from build123d import *

# Parameters (mm, degrees)
SKETCH1_W                = 76.2
SKETCH1_H                = 51
BOSS_EXTRUDE1_DEPTH      = 10
CHAMFER1_SIZE            = 2
BOSS_EXTRUDE2_DEPTH      = 38.1
BOSS_EXTRUDE2_DEPTH_BACK = 38.1
SKETCH2_W                = 32
SKETCH2_H                = 4.75
CUT_EXTRUDE1_DEPTH       = 32
FILLET1_R                = 13.5
SKETCH4_R                = 4
CUT_EXTRUDE2_DEPTH       = 10
BOSS_EXTRUDE4_START      = -9.1
SKETCH5_W                = 13.5
SKETCH5_H                = 18.25
BOSS_EXTRUDE4_DEPTH      = 8
BOSS_EXTRUDE5_START      = -67.1
SKETCH5_4_W              = 13.5
SKETCH5_4_H              = 18.25
BOSS_EXTRUDE5_DEPTH      = 8
FILLET2_R                = 11.5
BOSS_EXTRUDE6_START      = -9.64
SKETCH7_W                = 13.5
SKETCH7_H                = 10
BOSS_EXTRUDE6_DEPTH      = 6.5
BOSS_EXTRUDE7_START      = -32.36
SKETCH7_2_W              = 13.5
SKETCH7_2_H              = 10
BOSS_EXTRUDE7_DEPTH      = 6.65
FILLET3_R                = 11.5
CHAMFER3_SIZE            = 2
CHAMFER4_SIZE            = 1
SKETCH8_R                = 3.5
SKETCH8_R_2              = 1.8
CUT_EXTRUDE3_DEPTH       = 4.5
SKETCH8_4_R              = 1.8
CUT_EXTRUDE6_DEPTH       = 56.909391028
LPATTERN1_COUNT          = 2
LPATTERN1_PITCH          = 45
SKETCH10_6_R             = 1.8
CUT_EXTRUDE17_DEPTH      = 51.851352048
SKETCH10_R               = 3.5
SKETCH10_R_2             = 1.8
CUT_EXTRUDE11_DEPTH      = 3
SKETCH12_R               = 1.8
CUT_EXTRUDE13_DEPTH      = 56.909391028
SKETCH12_4_R             = 3.5
SKETCH12_4_R_2           = 1.8
CUT_EXTRUDE14_DEPTH      = 4.5
LPATTERN3_COUNT          = 2
LPATTERN3_PITCH          = 50
CUT_EXTRUDE18_DEPTH      = 71.73817429
CUT_EXTRUDE18_DEPTH_BACK = 2.5
SKETCH13_W               = 35
SKETCH13_H               = 12
FILLET4_R                = 8.5
CUT_EXTRUDE19_DEPTH      = 68.931380819
CUT_EXTRUDE19_DEPTH_BACK = 1.5
SKETCH14_R               = 3.5
SKETCH14_R_2             = 1.8
CUT_EXTRUDE20_DEPTH      = 68.931380875
CUT_EXTRUDE20_DEPTH_BACK = 68.931380875
SKETCH14_4_R             = 1.8


with BuildPart() as part:
    # Sketch1 → Boss-Extrude1 (new body)
    with BuildSketch(Plane.XY):
        Rectangle(SKETCH1_W, SKETCH1_H)
    extrude(amount=-BOSS_EXTRUDE1_DEPTH)

    # Chamfer1
    chamfer1_edges = [part.edges().sort_by_distance(p)[0] for p in [
        (-38.1, 25.5, -5),
        (38.1, 25.5, -5),
    ]]
    chamfer(chamfer1_edges, length=CHAMFER1_SIZE)

    # Sketch2 → Boss-Extrude2 (add, two sides: drawn at the far end of the back side and taken through both)
    with BuildSketch(Plane(origin=(0, 0, 0), x_dir=(0, 0, -1), z_dir=(1, 0, 0)).offset(-BOSS_EXTRUDE2_DEPTH_BACK)):
        with Locations((16, -23.125)):
            Rectangle(SKETCH2_W, SKETCH2_H)
    extrude(amount=BOSS_EXTRUDE2_DEPTH + BOSS_EXTRUDE2_DEPTH_BACK)

    # Sketch3 → Cut-Extrude1 (cut)
    with BuildSketch(Plane(origin=(0, -25.5, 0), x_dir=(-1, 0, 0), z_dir=(0, -1, 0))):
        Polygon((-7.67217, 0), (7.67217, 0), (9.268805, 5.32212), (-9.268805, 5.32212), align=None)
    extrude(amount=-CUT_EXTRUDE1_DEPTH, mode=Mode.SUBTRACT)

    # Fillet1
    fillet1_edges = [part.edges().sort_by_distance(p)[0] for p in [
        (0, -20.75, -10),
    ]]
    fillet(fillet1_edges, radius=FILLET1_R)

    # Sketch4 → Cut-Extrude2 (cut)
    with BuildSketch(Plane.XZ.offset(25.5)):
        with Locations((0, -11.5)):
            Circle(SKETCH4_R)
    extrude(amount=-CUT_EXTRUDE2_DEPTH, mode=Mode.SUBTRACT)

    # Sketch5 → Boss-Extrude4 (add)
    with BuildSketch(Plane(origin=(38.1, 0, 0), x_dir=(0, 0, -1), z_dir=(1, 0, 0)).offset(BOSS_EXTRUDE4_START)):
        with Locations((16.75, -11.625)):
            Rectangle(SKETCH5_W, SKETCH5_H)
    extrude(amount=-BOSS_EXTRUDE4_DEPTH)

    # Sketch5<4> → Boss-Extrude5 (add)
    with BuildSketch(Plane(origin=(38.1, 0, 0), x_dir=(0, 0, -1), z_dir=(1, 0, 0)).offset(BOSS_EXTRUDE5_START)):
        with Locations((16.75, -11.625)):
            Rectangle(SKETCH5_4_W, SKETCH5_4_H)
    extrude(amount=BOSS_EXTRUDE5_DEPTH)

    # Fillet2
    fillet2_edges = [part.edges().sort_by_distance(p)[0] for p in [
        (25, -2.5, -10),
        (-25, -2.5, -10),
    ]]
    fillet(fillet2_edges, radius=FILLET2_R)

    # Sketch7 → Boss-Extrude6 (add)
    with BuildSketch(Plane(origin=(21, 0, 0), x_dir=(0, 0, -1), z_dir=(1, 0, 0)).offset(BOSS_EXTRUDE6_START)):
        with Locations((16.75, 4)):
            Rectangle(SKETCH7_W, SKETCH7_H)
    extrude(amount=-BOSS_EXTRUDE6_DEPTH)

    # Sketch7<2> → Boss-Extrude7 (add)
    with BuildSketch(Plane(origin=(21, 0, 0), x_dir=(0, 0, -1), z_dir=(1, 0, 0)).offset(BOSS_EXTRUDE7_START)):
        with Locations((16.75, 4)):
            Rectangle(SKETCH7_2_W, SKETCH7_2_H)
    extrude(amount=BOSS_EXTRUDE7_DEPTH)

    # Fillet3
    # the kernel refuses this fillet: 11.5 mm, written as the material it adds along each edge
    with BuildSketch(Plane(origin=(11.36, -1, -10), x_dir=(0, -1, 0), z_dir=(-1, 0, 0))) as fillet3_piece_1:
        with BuildLine():
            CenterArc((FILLET3_R, -FILLET3_R), FILLET3_R, 90, 90)
            Line((0, -FILLET3_R), (0, 0))
            Line((0, 0), (FILLET3_R, 0))
        make_face()
    extrude(amount=6.5)
    with BuildSketch(Plane(origin=(11.36, -1, -10), x_dir=(0, -1, 0), z_dir=(-1, 0, 0))) as fillet3_piece_2_section:
        with BuildLine():
            CenterArc((FILLET3_R, -FILLET3_R), FILLET3_R, 90, 90)
            Line((0, -FILLET3_R), (0, 0))
            Line((0, 0), (FILLET3_R, 0))
        make_face()
    fillet3_piece_2 = extrude(amount=35.25, mode=Mode.PRIVATE)
    fillet3_piece_2 = split(fillet3_piece_2, bisect_by=Plane(origin=(-4.71, -3.603543814, -12.603543814), z_dir=(-1, 0, 0)), keep=Keep.TOP, mode=Mode.PRIVATE)
    fillet3_piece_2 = split(fillet3_piece_2, bisect_by=Plane(origin=(-11.36, -3.603543814, -12.603543814), z_dir=(1, 0, 0)), keep=Keep.TOP, mode=Mode.PRIVATE)
    add(fillet3_piece_2)
    with BuildSketch(Plane(origin=(-11.36, -1, -10), x_dir=(0, -1, 0), z_dir=(1, 0, 0))) as fillet3_piece_3:
        with BuildLine():
            CenterArc((FILLET3_R, FILLET3_R), FILLET3_R, 180, 90)
            Line((0, FILLET3_R), (0, 0))
            Line((0, 0), (FILLET3_R, 0))
        make_face()
    extrude(amount=6.65)
    with BuildSketch(Plane(origin=(-11.36, -1, -10), x_dir=(0, -1, 0), z_dir=(1, 0, 0))) as fillet3_piece_4_section:
        with BuildLine():
            CenterArc((FILLET3_R, FILLET3_R), FILLET3_R, 180, 90)
            Line((0, FILLET3_R), (0, 0))
            Line((0, 0), (FILLET3_R, 0))
        make_face()
    fillet3_piece_4 = extrude(amount=35.4, mode=Mode.PRIVATE)
    fillet3_piece_4 = split(fillet3_piece_4, bisect_by=Plane(origin=(11.36, -3.603543814, -12.603543814), z_dir=(-1, 0, 0)), keep=Keep.TOP, mode=Mode.PRIVATE)
    fillet3_piece_4 = split(fillet3_piece_4, bisect_by=Plane(origin=(4.86, -3.603543814, -12.603543814), z_dir=(1, 0, 0)), keep=Keep.TOP, mode=Mode.PRIVATE)
    add(fillet3_piece_4)

    # Chamfer3
    chamfer3_edges = [part.edges().sort_by_distance(p)[0] for p in [
        (38.1, -23.125, -32),
        (-38.1, -23.125, -32),
    ]]
    chamfer(chamfer3_edges, length=CHAMFER3_SIZE)

    # Chamfer4
    chamfer4_edges = [part.edges().sort_by_distance(p)[0] for p in [
        (-25, -2.5, -23.5),
        (8.11, 9, -23.5),
        (8.11, -1, -23.5),
        (0, 25.5, 0),
        (-8.035, -1, -23.5),
        (-8.035, 9, -23.5),
        (0, 25.5, -10),
        (0, -20.75, -32),
        (25, -2.5, -23.5),
    ]]
    chamfer(chamfer4_edges, length=CHAMFER4_SIZE)

    # Sketch8 → Cut-Extrude3 (cut)
    with BuildSketch(Plane.XY):
        with Locations((-30.63, 21.5)):
            Circle(SKETCH8_R)
        with Locations((-30.63, 21.5)):
            Circle(SKETCH8_R_2, mode=Mode.SUBTRACT)
    cut_extrude3 = extrude(amount=-CUT_EXTRUDE3_DEPTH, mode=Mode.SUBTRACT)

    # Sketch8<4> → Cut-Extrude6 (cut, through all)
    with BuildSketch(Plane.XY):
        with Locations((-30.63, 21.5)):
            Circle(SKETCH8_4_R)
    cut_extrude6 = extrude(amount=-CUT_EXTRUDE6_DEPTH, mode=Mode.SUBTRACT)

    # LPattern1: Cut-Extrude3, Cut-Extrude6 ×2
    with Locations(*[(i * LPATTERN1_PITCH, 0, 0) for i in range(1, LPATTERN1_COUNT)]):
        add(cut_extrude3, mode=Mode.SUBTRACT)
        add(cut_extrude6, mode=Mode.SUBTRACT)

    # Sketch10<6> → Cut-Extrude17 (cut, through all)
    with BuildSketch(Plane.XY.offset(-10)):
        with Locations(Location((-16.6, 6.5, 0), (0, 0, 180))):
            Circle(SKETCH10_6_R)
        with Locations(Location((15.4, 6.5, 0), (0, 0, 180))):
            Circle(SKETCH10_6_R)
    extrude(amount=CUT_EXTRUDE17_DEPTH, mode=Mode.SUBTRACT)

    # Sketch10 → Cut-Extrude11 (cut)
    # profile 1 of 2: a face of its own
    with BuildSketch(Plane.XY.offset(-10)):
        with Locations(Location((-16.6, 6.5, 0), (0, 0, 180))):
            Circle(SKETCH10_R)
        with Locations(Location((-16.6, 6.5, 0), (0, 0, 180))):
            Circle(SKETCH10_R_2, mode=Mode.SUBTRACT)
    # profile 2 of 2: a face of its own
    with BuildSketch(Plane.XY.offset(-10)):
        with Locations(Location((15.4, 6.5, 0), (0, 0, 180))):
            Circle(SKETCH10_R)
        with Locations(Location((15.4, 6.5, 0), (0, 0, 180))):
            Circle(SKETCH10_R_2, mode=Mode.SUBTRACT)
    extrude(amount=CUT_EXTRUDE11_DEPTH, mode=Mode.SUBTRACT)

    # Sketch12 → Cut-Extrude13 (cut, through all)
    with BuildSketch(Plane.XY):
        with Locations((-25, -8.5)):
            Circle(SKETCH12_R)
    cut_extrude13 = extrude(amount=-CUT_EXTRUDE13_DEPTH, mode=Mode.SUBTRACT)

    # Sketch12<4> → Cut-Extrude14 (cut)
    with BuildSketch(Plane.XY):
        with Locations((-25, -8.5)):
            Circle(SKETCH12_4_R)
        with Locations((-25, -8.5)):
            Circle(SKETCH12_4_R_2, mode=Mode.SUBTRACT)
    cut_extrude14 = extrude(amount=-CUT_EXTRUDE14_DEPTH, mode=Mode.SUBTRACT)

    # LPattern3: Cut-Extrude13, Cut-Extrude14 ×2
    with Locations(*[(i * LPATTERN3_PITCH, 0, 0) for i in range(1, LPATTERN3_COUNT)]):
        add(cut_extrude13, mode=Mode.SUBTRACT)
        add(cut_extrude14, mode=Mode.SUBTRACT)

    # Sketch13 → Cut-Extrude18 (cut, two sides: drawn at the far end of the back side and taken through both)
    with BuildSketch(Plane(origin=(0, -20.75, 5.592775926), x_dir=(1, 0, 0), z_dir=(0, 1, 0)).offset(-CUT_EXTRUDE18_DEPTH_BACK)):
        with Locations((0, 31.592775926)):
            Rectangle(SKETCH13_W, SKETCH13_H)
    extrude(amount=CUT_EXTRUDE18_DEPTH + CUT_EXTRUDE18_DEPTH_BACK, mode=Mode.SUBTRACT)

    # Fillet4
    # the kernel refuses this fillet: 8.5 mm, written as the material it adds along each edge
    with BuildSketch(Plane(origin=(33.619877511, -23.25, -20), x_dir=(0, 0, -1), z_dir=(-1, 0, 0))) as fillet4_piece_1:
        with BuildLine():
            CenterArc((6.447951004, -8.5), FILLET4_R, 90, 49.339390538)
            Line((0, -2.96159519), (-0.12895902, -2.850827093))
            ThreePointArc((-0.12895902, -2.850827093), (-0.17, -1.480797595), (-0.17, 0))
            Line((-0.17, 0), (0, 0.17))
            Line((0, 0.17), (6.447951004, 0.17))
            Line((6.447951004, 0.17), (6.447951004, 0))
        make_face()
    extrude(amount=67.239755022)

    # Sketch14 → Cut-Extrude19 (cut, two sides: drawn at the far end of the back side and taken through both)
    # profile 1 of 2: a face of its own
    with BuildSketch(Plane(origin=(0, -20.75, 0), x_dir=(1, 0, 0), z_dir=(0, 1, 0)).offset(-CUT_EXTRUDE19_DEPTH_BACK)):
        with Locations(Location((-33.55, 17, 0), (0, 0, 90))):
            Circle(SKETCH14_R)
        with Locations(Location((-33.55, 17, 0), (0, 0, 90))):
            Circle(SKETCH14_R_2, mode=Mode.SUBTRACT)
    # profile 2 of 2: a face of its own
    with BuildSketch(Plane(origin=(0, -20.75, 0), x_dir=(1, 0, 0), z_dir=(0, 1, 0)).offset(-CUT_EXTRUDE19_DEPTH_BACK)):
        with Locations(Location((33.55, 17, 0), (0, 0, 90))):
            Circle(SKETCH14_R)
        with Locations(Location((33.55, 17, 0), (0, 0, 90))):
            Circle(SKETCH14_R_2, mode=Mode.SUBTRACT)
    extrude(amount=CUT_EXTRUDE19_DEPTH + CUT_EXTRUDE19_DEPTH_BACK, mode=Mode.SUBTRACT)

    # Sketch14<4> → Cut-Extrude20 (cut, two sides: drawn at the far end of the back side and taken through both)
    with BuildSketch(Plane(origin=(0, -20.75, 0), x_dir=(1, 0, 0), z_dir=(0, 1, 0)).offset(-CUT_EXTRUDE20_DEPTH_BACK)):
        with Locations(Location((33.55, 17, 0), (0, 0, 270))):
            Circle(SKETCH14_4_R)
        with Locations(Location((-33.55, 17, 0), (0, 0, 270))):
            Circle(SKETCH14_4_R)
    extrude(amount=CUT_EXTRUDE20_DEPTH + CUT_EXTRUDE20_DEPTH_BACK, mode=Mode.SUBTRACT)


solid = part.part
Could you check a few things on this model? Use its own coordinates, in mm. A direction names the side the tool comes from. Give positions to 0.01 mm unless a question says otherwise; leave off trailing zeros. Write each loop counter-clockwise with the first axis right and the second up, starting at its lowest first coordinate (ties: lowest second). Pieces come first, ordered by that corner, then holes. Notation, with made-up numbers: (56, -3.5) - (110, -3.5) arc R22 ccw to (110, 33.5) - close; hole circle Ø9 at (-22.75, 80). An arc over 180 degrees is marked (long way). Use CSV: the item, a comma, the result in double quotes. Start each with the question number.
Item 1: For faces 1 (the face through (-34, -22.25, -15)), 2 (the face through (16.159, 9.917, -8.521)), 3 (the face through (8.482, -9.724, -2.698)), 4 (the face through (8, 4, -20)), which set-ups out of +Z, -Z, +X, -X, +Y, -Y let a thin tool reach every point of the face, with its end or its side?
Item 2: I want a section at D-D, the plane y = 15. Please give me the cut outline in (x, z), then the cut area to 3 significant figures.
Item 3: I want a section at B-B, the plane z = -25. Please give me the cut outline in (x, y), then the cut area to 3 significant figures.
Item 4: I want a section at C-C, the plane x = 25. Please give me the cut outline in (y, z).
Item 5: If I drill on line 1 along Z through (x, y) = (-33.55, -23.15); line 2 along Y through (x, z) = (-30.63, -7.9); line 3 along X through (y, z) = (-13, -17), over which ranges is the centre line in solid material (lowest first)?
Item 6: If we mould it in two halves opening along Y, with no side actions, what happens to faces 5 (the face through (-29, 20, -4.5)), 6 (the face through (37.1, 24.5, -4.9)), 7 (the face through (-1, 12, -10))? For each: pulls with the +Y half, pulls with the -Y half, needs draft (parallel to the pull), parting line crosses it, or undercut.
Item 7: I'm going to push flat-ended pins straight in: pin 1 (12 mm diameter, centred on y = 4.5, z = -18.5, fed in from +X); pin 2 (4 mm diameter, centred on y = -10, z = -20, fed in from +X); pin 3 (7.5 mm diameter, centred on x = 34.5, z = -17.5, fed in from +Y). Where does each tip first touch, or does it pass through?
Item 8: I want a section at A-A, the plane x = -16.6. Please give me the cut outline in (y, z).
Findings:
1,face 1,"+Y"
1,face 2,"-Z"
1,face 3,"-Y"
1,face 4,"-Z, +X, -X, +Y"
2,outline,"(-38.1, -10) - (38.1, -10) - (38.1, 0) - (-38.1, 0) - close"
2,area,"762 mm2"
3,outline,"(-38.1, -25.5) - (38.1, -25.5) - (38.1, -20.75) - (17.5, -20.75) - (17.5, -23.13) - (-17.5, -23.13) - (-17.5, -20.75) - (-38.1, -20.75) - close"
3,area,"279 mm2"
4,outline,"(-25.5, -32) - (-21.75, -32) - (-20.75, -31) - (-20.75, -23.5) - (-10.3, -23.5) - (-10.3, -4.5) - (-12, -4.5) - (-12, 0) - (-25.5, 0) - close; (-6.7, -23.5) - (-3.5, -23.5) - (-2.5, -22.5) - (-2.5, -21.5) arc R11.5 cw to (9, -10) - (24.5, -10) - (25.5, -9) - (25.5, -1) - (24.5, 0) - (-5, 0) - (-5, -4.5) - (-6.7, -4.5) - close"
5,line 1,"z = -32 to -18.8, -15.2 to 0"
5,line 2,"y = -25.5 to 19.7, 23.3 to 25.5"
5,line 3,"x = -29 to -21, 21 to 29"
6,face 5,"undercut"
6,face 6,"pulls with the +Y half"
6,face 7,"needs draft"
7,pin 1,"stops at x = 11.36"
7,pin 2,"stops at x = 29"
7,pin 3,"stops at y = -16.61"
8,outline,"(-25.5, -32) - (-23.25, -32) - (-23.25, -26.45) arc R8.5 cw to (-20.29, -20) arc R13.5 cw to (-7.25, -10) - (3, -10) - (3, -7) - (4.7, -7) - (4.7, 0) - (-25.5, 0) - close; (8.3, -7) - (10, -7) - (10, -10) - (24.5, -10) - (25.5, -9) - (25.5, -1) - (24.5, 0) - (8.3, 0) - close"
